Can you work these out from the drawing? Everything is in mm from the part's minimum corner. A direction names the side the tool comes from. Round coordinates to 2 decimals unless told otherwise and drop trailing zeros. Loops run counter-clockwise (first coordinate to the right, second up) from the corner with the lowest first, then second, coordinate; pieces in that order, holes last. Notation, with made-up numbers: M 70.25,41 L 104.25,41 A11 ccw 104.25,61 Z; hole C 18,79 d10. An arc over 180 degrees is marked long. Answer in a Markdown table with one row per item.
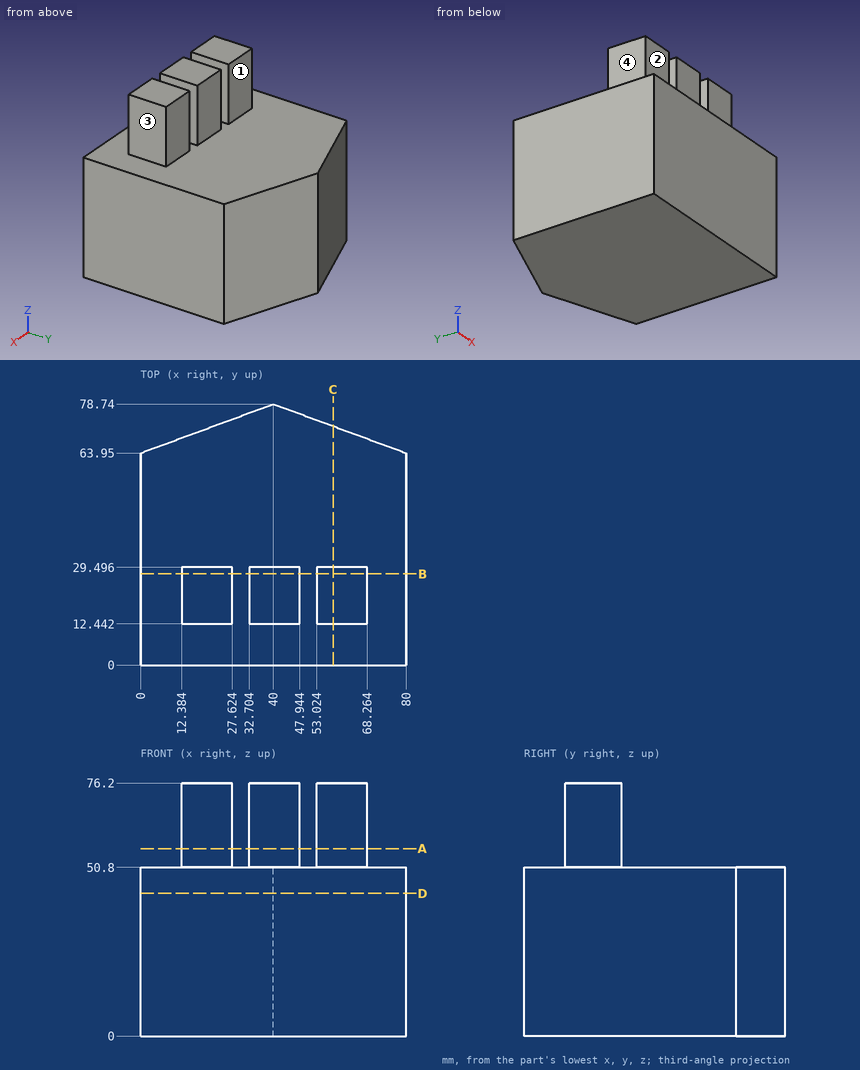
1) I need wall thicknesses on line 1 (X direction, y = 24, z = 68.5) (1 decimal); line 2 (Z direction, x = 38, y = 59); line 3 (Y direction, x = 42, z = 33.5). Which ranges of each line are inside material? Lowest first, please.
Computed:
| item | result |
|---|---|
| line 1 | x = 12.4 to 27.6, 32.7 to 47.9, 53 to 68.3 |
| line 2 | z = 0 to 50.8 |
| line 3 | y = 0 to 78 |
2) I want a section at C-C, the plane x = 58. Please give me the cut outline in (y, z) (1 decimal).
Computed:
| item | result |
|---|---|
| outline | M 0,0 L 72.1,0 L 72.1,50.8 L 29.5,50.8 L 29.5,76.2 L 12.4,76.2 L 12.4,50.8 L 0,50.8 Z |
3) I want a section at B-B, the plane y = 27.5. Please give me the cut outline in (x, z) (1 decimal).
Computed:
| item | result |
|---|---|
| outline | M 0,0 L 80,0 L 80,50.8 L 68.3,50.8 L 68.3,76.2 L 53,76.2 L 53,50.8 L 47.9,50.8 L 47.9,76.2 L 32.7,76.2 L 32.7,50.8 L 27.6,50.8 L 27.6,76.2 L 12.4,76.2 L 12.4,50.8 L 0,50.8 Z |
4) I want a section at A-A, the plane z = 56.5. Please give me the cut outline in (x, y) (1 decimal), plus the area to 3 significant figures.
Computed:
| item | result |
|---|---|
| outline | M 12.4,12.4 L 27.6,12.4 L 27.6,29.5 L 12.4,29.5 Z; M 32.7,12.4 L 47.9,12.4 L 47.9,29.5 L 32.7,29.5 Z; M 53,12.4 L 68.3,12.4 L 68.3,29.5 L 53,29.5 Z |
| area | 780 mm² |
5) Will these pins go through, and if not, where does the flat tip stop? P1, Ø7.5, axis at x = 39, z = 60, coming from the -Y side; P2, Ø19, axis at y = 20, z = 59.5, coming from the +X side; P3, Ø12, axis at x = 49.5, z = 64.5, coming from the +Y side; P4, Ø13.5, axis at y = 21.5, z = 65, coming from the +X side.
Computed:
| item | result |
|---|---|
| P1 | stops at y = 12.44 |
| P2 | stops at x = 80 |
| P3 | stops at y = 29.5 |
| P4 | stops at x = 68.26 |
6) Which directions (+Z, -Z, +X, -X, +Y, -Y) give clear straight access to the entire face, cutting with the end or side of a thin tool? Please do the marked faces 1, 2, 3 and 4.
Computed:
| item | result |
|---|---|
| face 1 | +Z, +X, -X, +Y |
| face 2 | +Z, +X, -X, -Y |
| face 3 | +Z, +X, +Y, -Y |
| face 4 | +Z, -X, +Y, -Y |
7) I want a section at D-D, the plane z = 43. Please give me the cut outline in (x, y).
Computed:
| item | result |
|---|---|
| outline | M 0,0 L 80,0 L 80,63.95 L 40,78.74 L 0,63.95 Z |
